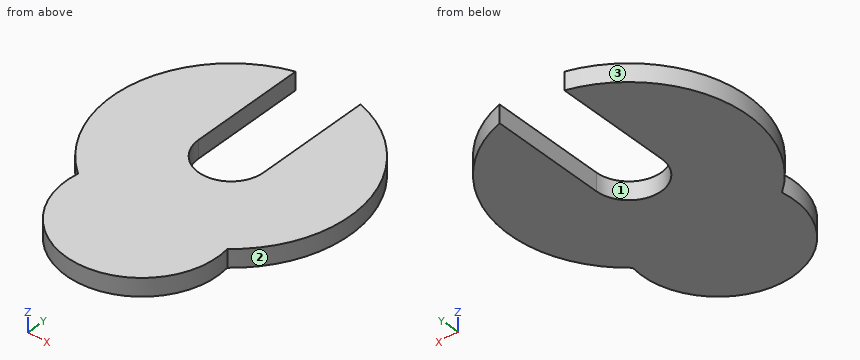
from build123d import *

# Parameters (mm, degrees)
F1_DEPTH = 1.65


with BuildPart() as f1:
    # F0 (on Top) → F1 (new body)
    with BuildSketch(Plane.XY):
        with BuildLine():
            Line((-3, 0), (-3, 10.583005))
            ThreePointArc((-3, 10.583005), (-10.778469, 2.196498), (-6.902109, -8.565097))
            ThreePointArc((-6.902109, -8.565097), (0, -11), (6.902109, -8.565097))
            ThreePointArc((6.902109, -8.565097), (10.778469, 2.196498), (3, 10.583005))
            Line((3, 10.583005), (3, 0))
            ThreePointArc((3, 0), (0, -3), (-3, 0))
        make_face()
        with BuildLine():
            ThreePointArc((6.902109, -8.565097), (0, -11), (-6.902109, -8.565097))
            ThreePointArc((-6.902109, -8.565097), (0, -16.731671), (6.902109, -8.565097))
        make_face()
    extrude(amount=F1_DEPTH)


solid = f1.part
Model file for the job. Use its own axes, mm. Face numbers are marked on the shaded views. Give positions to 0.01 mm unless a question says otherwise; leave off trailing zeros. Loops run counter-clockwise (first coordinate to the right, second up) from the corner with the lowest first, then second, coordinate; pieces in that order, holes last. Notation, with made-up numbers: (59.25, 19) -> (82.25, 19) arc R28 ccw to (82.25, 57) -> close; hole circle Ø7 at (15, 14.25). An arc over 180 degrees is marked (long way). Use a Markdown table: item, result. Add a question column.
(1) Wall check: line 1 along X through (y, z) = (-9.5, 0.35); line 2 along X through (y, z) = (1.5, 0.25); line 3 along X through (y, z) = (8.5, 1.15). Give the ranges that are in metal, low to high.
(2) Drop flat-ended pins along their axis: pin 1 Ø0.5 at (y, z) = (7.5, 1) entering from -X; pin 2 Ø4 at (x, y) = (-8.5, -13) entering from +Z. Give the stop position or say it passes through.
(3) Slice it at D-D on y = -6. List the corners of the cut face in (x, z), and give its area (3 significant figures).
(4) Slice it at B-B on z = 0.95. List the corners of the cut face in (x, y), and give its area (3 significant figures).
(5) Slice it at C-C on x = 0. List the corners of the cut face in (y, z), and give its area (3 significant figures).
(6) Mould opens along X. For the marked faces 1, 2 and 3 say: +X half, -X half, draft (parallel to the pull), parting line (faces both ways), or undercut.
(7) Slice it at A-A on y = 3. List the corners of the cut face in (x, z), and give its area (3 significant figures).
Filled sheet:
| question | item | result |
|---|---|---|
| 1 | line 1 | -7 to 7 |
| 1 | line 2 | -10.9 to -3, 3 to 10.9 |
| 1 | line 3 | -6.98 to -3, 3 to 6.98 |
| 2 | pin 1 | x = -8.27 |
| 2 | pin 2 | through |
| 3 | outline | (-9.22, 0) -> (9.22, 0) -> (9.22, 1.65) -> (-9.22, 1.65) -> close |
| 3 | area | 30.4 mm2 |
| 4 | outline | (-6.9, -8.57) arc R7 ccw (long way) to (6.9, -8.57) arc R11 ccw to (3, 10.58) -> (3, 0) arc R3 cw to (-3, 0) -> (-3, 10.58) arc R11 ccw to start |
| 4 | area | 371 mm2 |
| 5 | outline | (-16.73, 0) -> (-3, 0) -> (-3, 1.65) -> (-16.73, 1.65) -> close |
| 5 | area | 22.7 mm2 |
| 6 | face 1 | undercut |
| 6 | face 2 | +X half |
| 6 | face 3 | -X half |
| 7 | outline | (-10.58, 0) -> (-3, 0) -> (-3, 1.65) -> (-10.58, 1.65) -> close; (3, 0) -> (10.58, 0) -> (10.58, 1.65) -> (3, 1.65) -> close |
| 7 | area | 25.0 mm2 |
